Work out the finished part from the listing and answer in its coordinate system (mm). Coordinates: 2 decimals unless noted, no trailing zeros. Write each loop counter-clockwise with the first axis right and the second up, starting at its lowest first coordinate (ties: lowest second). Pieces come first, ordered by that corner, then holes. Notation, with made-up numbers: M -28,34 L -19,34 A17 ccw -19,62 Z; hole C -30.5,63.5 d5. An arc over 180 degrees is marked long. Answer as CSV lines item,"result". Start each with the question number.
(1) Find the intervals of material crossed by L1, parallel to Y at x = 21, z = 2.75; L2, parallel to Y at x = -3, z = 2.05; L3, parallel to X at y = 94.5, z = 1.05, in increasing order. Write a range as [from, to].
(2) A cutting plane is placed at A-A on x = 5. Give the vertices of the cut face in (y, z), then the cut area to 3 significant figures.
(3) A cutting plane is placed at B-B on y = 30.5. Give the vertices of the cut face in (x, z), then the cut area to 3 significant figures.
(4) Flat-ended cylindrical pins translate along their axes: P1, Ø0.9, axis at x = -49, z = 2, coming from the -Y side; P2, Ø0.9, axis at y = 199, z = 1, coming from the -X side; P3, Ø0.9, axis at x = 49, z = 1, coming from the +Y side; P4, Ø2, axis at x = 24.5, y = 56, coming from the -Z side. Find the tip coordinate at first contact, or state that the pin passes through.
from build123d import *

# Parameters (mm, degrees)
SKETCH1_W           = 100
SKETCH1_H           = 400
BOSS_EXTRUDE1_DEPTH = 3
SKETCH2_W           = 20
SKETCH2_H           = 3
CUT_EXTRUDE1_DEPTH  = 3
SKETCH4_W           = 3
SKETCH4_H           = 47
SKETCH4_H_2         = 50
CUT_EXTRUDE2_DEPTH  = 3
CAVITY1_START       = 97.807385879
CAVITY1_OUTLINE_W   = 60
CAVITY1_OUTLINE_H   = 3
CAVITY1_DEPTH       = 3


# Read off the part's stored shape, not the designer's step: Cavity1
with BuildPart() as part:
    # Sketch1 → Boss-Extrude1 (new body)
    with BuildSketch(Plane.XY):
        Rectangle(SKETCH1_W, SKETCH1_H)
    extrude(amount=BOSS_EXTRUDE1_DEPTH)

    # Sketch2 → Cut-Extrude1 (cut)
    with BuildSketch(Plane.XY.offset(3)):
        with Locations((-40, -198.5)):
            Rectangle(SKETCH2_W, SKETCH2_H)
        with Locations((0, -198.5)):
            Rectangle(SKETCH2_W, SKETCH2_H)
        with Locations((40, -198.5)):
            Rectangle(SKETCH2_W, SKETCH2_H)
        with Locations((40, 198.5)):
            Rectangle(SKETCH2_W, SKETCH2_H)
        with Locations((0, 198.5)):
            Rectangle(SKETCH2_W, SKETCH2_H)
        with Locations((-40, 198.5)):
            Rectangle(SKETCH2_W, SKETCH2_H)
    extrude(amount=-CUT_EXTRUDE1_DEPTH, mode=Mode.SUBTRACT)

    # Sketch4 → Cut-Extrude2 (cut)
    with BuildSketch(Plane(origin=(0, 0, 0), x_dir=(-1, 0, 0), z_dir=(0, 0, -1))):
        with Locations((-48.5, 173.5)):
            Rectangle(SKETCH4_W, SKETCH4_H)
        with Locations((-48.5, 25)):
            Rectangle(SKETCH4_W, SKETCH4_H_2)
        with Locations((-48.5, -72)):
            Rectangle(SKETCH4_W, SKETCH4_H_2)
        with Locations((-48.5, -172)):
            Rectangle(SKETCH4_W, SKETCH4_H_2)
        with Locations((48.5, -172)):
            Rectangle(SKETCH4_W, SKETCH4_H_2)
        with Locations((48.5, -72)):
            Rectangle(SKETCH4_W, SKETCH4_H_2)
        with Locations((48.5, 25)):
            Rectangle(SKETCH4_W, SKETCH4_H_2)
        with Locations((48.5, 173.5)):
            Rectangle(SKETCH4_W, SKETCH4_H)
        with Locations((48.5, 100)):
            Rectangle(SKETCH4_W, SKETCH4_H_2)
        with Locations((-48.5, 100)):
            Rectangle(SKETCH4_W, SKETCH4_H_2)
    extrude(amount=-CUT_EXTRUDE2_DEPTH, mode=Mode.SUBTRACT)

    # Cavity1 outline → Cavity1 (cut)
    with BuildSketch(Plane(origin=(0, 0, 0), x_dir=(1, 0, 0), z_dir=(0, 1, 0)).offset(CAVITY1_START)):
        with Locations((0, -1.5)):
            Rectangle(CAVITY1_OUTLINE_W, CAVITY1_OUTLINE_H)
    extrude(amount=CAVITY1_DEPTH, mode=Mode.SUBTRACT)


solid = part.part
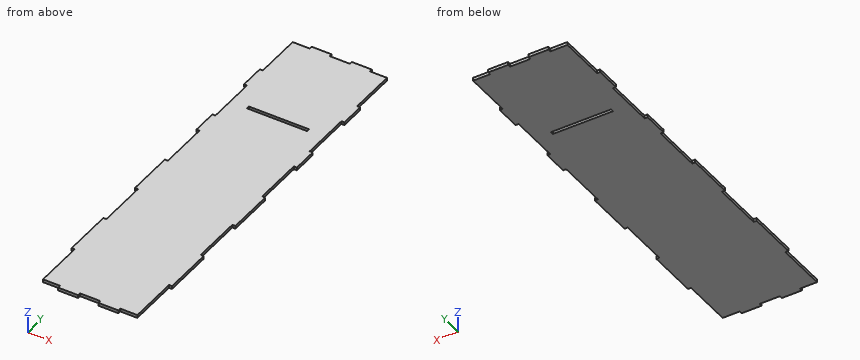
Here are the results:
1,L1,"y = [-200, 97.81], [100.81, 200]"
1,L2,"y = [-197, 97.81], [100.81, 197]"
1,L3,"x = [-47, 47]"
2,outline,"M -197,0 L 97.81,0 L 97.81,3 L -197,3 Z; M 100.81,0 L 197,0 L 197,3 L 100.81,3 Z"
2,area,"1,170 mm^2"
3,outline,"M -47,0 L 47,0 L 47,3 L -47,3 Z"
3,area,"282 mm^2"
4,P1,"stops at y = -147"
4,P2,"stops at x = -30"
4,P3,"stops at y = 150"
4,P4,"stops at z = 0"
